Could you check a few things on this model? Use its own coordinates, in mm. A direction names the side the tool comes from. Give positions to 0.01 mm unless a question says otherwise; leave off trailing zeros. Write each loop counter-clockwise with the first axis right and the second up, starting at its lowest first coordinate (ties: lowest second). Pieces come first, ordered by that corner, then holes. Notation, with made-up numbers: (14, -20) - (34, -20) arc R8 ccw to (34, -6) - close; hole circle Ø6 at (-15.75, 62). An arc over 180 degrees is marked (long way). Answer as CSV lines item,"result". Start each with the question number.
Q1. Imagine slicing it at D-D on x = 0. List the corners of the cut face in (y, z) for me.
Q2. Imagine slicing it at A-A on y = 18. List the corners of the cut face in (x, z) for me, and give its area (3 significant figures).
Q3. Imagine slicing it at C-C on x = 7.5. List the corners of the cut face in (y, z) for me.
Q4. Will these pins go through, and if not, where does the flat tip stop? pin 1 Ø2 at (x, z) = (-21, 3.5) entering from +Y; pin 2 Ø10.5 at (x, z) = (-2.5, 2.5) entering from +Y; pin 3 Ø1.5 at (y, z) = (45.25, 7.35) entering from +X; pin 4 Ø2 at (x, z) = (-20, -2.5) entering from +Y.
Q5. We'd pull the mould along X, two halves only. Please class faces 1 (the face through (21.35, 28, 0)), 2 (the face through (-21.35, 29, 0)), 3 (the face through (-20.336, 36.647, 0.055)), 4 (the face through (-14, -1, 0)): pulls with the +X half, pulls with the -X half, needs draft (parallel to the pull), parting line crosses it, or undercut.
Q6. If I drill on line 1 along X through (y, z) = (49, 9); line 2 along Z through (x, y) = (7.5, -0.65); line 3 along X through (y, z) = (-1.2, 5), over which ranges is the centre line in solid material (lowest first)?
Q7. Imagine slicing it at B-B on x = -10. List the corners of the cut face in (y, z) for me.
Q8. On a 3-axis mill with a long thin cutter (end or side, diameter ignored), from which of +Z, -Z, +X, -X, +Y, -Y can I reach the whole of each face in a straight line? I mean faces 5 (the face through (-20.336, 33.843, 6.145)), 6 (the face through (-2.55, -0.99, 2.5)), 7 (the face through (4, 0, -2)). Say none if no direction works.
```python
from build123d import *

# Parameters (mm, degrees)
CROQUIS2_W                  = 152.7
CROQUIS2_H                  = 21
BRIDA_BASE1_DEPTH           = 2
PLIEGUE_START               = -10.5
PLIEGUE_CROQUIZADO1_DEPTH   = 21
PLIEGUE_CROQUIZADO1_2_DEPTH = 21
CROQUIS8_R                  = 1.25
CROQUIS8_R_2                = 3
CORTAR_EXTRUIR1_DEPTH       = 72.000595879
CROQUIS9_R                  = 1.5
CORTAR_EXTRUIR2_DEPTH       = 2


# Read off the part's stored shape, not the designer's step: Pliegue croquizado1
# Sheet-metal steps are written as plain solids
with BuildPart() as part:
    # Croquis2 → Brida base1 (new body)
    with BuildSketch(Plane(origin=(0, 0, 0), x_dir=(1, 0, 0), z_dir=(0, 1, 0))):
        Rectangle(CROQUIS2_W, CROQUIS2_H)
    extrude(amount=-BRIDA_BASE1_DEPTH)

    # Pliegue croquizado1 outline → Pliegue croquizado1 (cut)
    with BuildSketch(Plane.XY.offset(PLIEGUE_START)):
        with BuildLine():
            Line((-76.35, -2), (-18.6134, -2))
            ThreePointArc((-18.6134, -2), (-20.267667209, -1.443395312), (-21.249002398, 0))
            Line((-21.249002398, 0), (-76.35, 0))
            Line((-76.35, 0), (-76.35, -2))
        make_face()
        with BuildLine():
            ThreePointArc((21.249002398, 0), (20.267667209, -1.443395312), (18.6134, -2))
            Line((18.6134, -2), (76.35, -2))
            Line((76.35, -2), (76.35, 0))
            Line((76.35, 0), (21.249002398, 0))
        make_face()
    extrude(amount=PLIEGUE_CROQUIZADO1_DEPTH, mode=Mode.SUBTRACT)

    # Pliegue croquizado1 2 outline → Pliegue croquizado1 2 (add)
    with BuildSketch(Plane.XY.offset(PLIEGUE_START)):
        with BuildLine():
            ThreePointArc((-21.35, 0.7366), (-21.324633029, 0.364854094), (-21.249002398, 0))
            Line((-21.249002398, 0), (-18.6134, 0))
            ThreePointArc((-18.6134, 0), (-19.134254855, 0.215745145), (-19.35, 0.7366))
            Line((-19.35, 0.7366), (-19.35, 55.745355099))
            Line((-19.35, 55.745355099), (-21.35, 55.745355099))
            Line((-21.35, 55.745355099), (-21.35, 0.7366))
        make_face()
        with BuildLine():
            Line((18.6134, 0), (21.249002398, 0))
            ThreePointArc((21.249002398, 0), (21.324633029, 0.364854094), (21.35, 0.7366))
            Line((21.35, 0.7366), (21.35, 55.745355099))
            Line((21.35, 55.745355099), (19.35, 55.745355099))
            Line((19.35, 55.745355099), (19.35, 0.7366))
            ThreePointArc((19.35, 0.7366), (19.134254855, 0.215745145), (18.6134, 0))
        make_face()
    extrude(amount=PLIEGUE_CROQUIZADO1_2_DEPTH)

    # Croquis8 → Cortar-Extruir1 (cut, through all)
    with BuildSketch(Plane(origin=(21.35, 0, 0), x_dir=(0, 0, -1), z_dir=(1, 0, 0))):
        with BuildLine():
            Line((-7, 8.745355099), (-7, 31.745355099))
            ThreePointArc((-7, 31.745355099), (-6.121320344, 33.866675442), (-4, 34.745355099))
            Line((-4, 34.745355099), (-2, 34.745355099))
            Line((-2, 34.745355099), (-2, 5.745355099))
            Line((-2, 5.745355099), (-4, 5.745355099))
            ThreePointArc((-4, 5.745355099), (-6.121320344, 6.624034755), (-7, 8.745355099))
        make_face()
        with BuildLine():
            Line((2, 5.745355099), (4, 5.745355099))
            ThreePointArc((4, 5.745355099), (6.121320344, 6.624034755), (7, 8.745355099))
            Line((7, 8.745355099), (7, 31.745355099))
            ThreePointArc((7, 31.745355099), (6.121320344, 33.866675442), (4, 34.745355099))
            Line((4, 34.745355099), (2, 34.745355099))
            Line((2, 34.745355099), (2, 5.745355099))
        make_face()
        with BuildLine():
            ThreePointArc((0, 55.745355099), (7.424621202, 52.669976301), (10.5, 45.245355099))
            Line((10.5, 45.245355099), (10.5, 55.745355099))
            Line((10.5, 55.745355099), (0, 55.745355099))
        make_face()
        with BuildLine():
            ThreePointArc((-10.5, 45.245355099), (-7.424621202, 52.669976301), (0, 55.745355099))
            Line((0, 55.745355099), (-10.5, 55.745355099))
            Line((-10.5, 55.745355099), (-10.5, 45.245355099))
        make_face()
        with Locations(Location((-7.35, 45.245355099, 0), (0, 0, 90))):
            Circle(CROQUIS8_R)
        with Locations(Location((0, 37.895355099, 0), (0, 0, 90))):
            Circle(CROQUIS8_R)
        with Locations(Location((7.35, 45.245355099, 0), (0, 0, 90))):
            Circle(CROQUIS8_R)
        with Locations(Location((0, 52.595355099, 0), (0, 0, 90))):
            Circle(CROQUIS8_R)
        with Locations(Location((0, 45.245355099, 0), (0, 0, 90))):
            Circle(CROQUIS8_R_2)
    extrude(amount=-CORTAR_EXTRUIR1_DEPTH, mode=Mode.SUBTRACT)

    # Croquis9 → Cortar-Extruir2 (cut)
    with BuildSketch(Plane(origin=(0, 0, 0), x_dir=(1, 0, 0), z_dir=(0, 1, 0))):
        with Locations(Location((-7.5, 5, 0), (0, 0, 270))):
            Circle(CROQUIS9_R)
        with Locations(Location((-7.5, -5, 0), (0, 0, 270))):
            Circle(CROQUIS9_R)
        with Locations(Location((7.5, -5, 0), (0, 0, 90))):
            Circle(CROQUIS9_R)
        with Locations(Location((7.5, 5, 0), (0, 0, 90))):
            Circle(CROQUIS9_R)
        with BuildLine():
            Line((-5, 1.5), (-12.5, 1.5))
            ThreePointArc((-12.5, 1.5), (-14, 0), (-12.5, -1.5))
            Line((-12.5, -1.5), (-5, -1.5))
            ThreePointArc((-5, -1.5), (-2.525126266, -2.525126266), (-1.5, -5))
            ThreePointArc((-1.5, -5), (0, -6.5), (1.5, -5))
            ThreePointArc((1.5, -5), (2.525126266, -2.525126266), (5, -1.5))
            Line((5, -1.5), (12.5, -1.5))
            ThreePointArc((12.5, -1.5), (14, 0), (12.5, 1.5))
            Line((12.5, 1.5), (5, 1.5))
            ThreePointArc((5, 1.5), (2.525126266, 2.525126266), (1.5, 5))
            ThreePointArc((1.5, 5), (0, 6.5), (-1.5, 5))
            ThreePointArc((-1.5, 5), (-2.525126266, 2.525126266), (-5, 1.5))
        make_face()
    extrude(amount=-CORTAR_EXTRUIR2_DEPTH, mode=Mode.SUBTRACT)


solid = part.part
```
Conclusion:
1,outline,"(-2, -10.5) - (0, -10.5) - (0, -6.5) - (-2, -6.5) - close; (-2, 6.5) - (0, 6.5) - (0, 10.5) - (-2, 10.5) - close"
2,outline,"(-21.35, -10.5) - (-19.35, -10.5) - (-19.35, -7) - (-21.35, -7) - close; (-21.35, -2) - (-19.35, -2) - (-19.35, 2) - (-21.35, 2) - close; (-21.35, 7) - (-19.35, 7) - (-19.35, 10.5) - (-21.35, 10.5) - close; (19.35, -10.5) - (21.35, -10.5) - (21.35, -7) - (19.35, -7) - close; (19.35, -2) - (21.35, -2) - (21.35, 2) - (19.35, 2) - close; (19.35, 7) - (21.35, 7) - (21.35, 10.5) - (19.35, 10.5) - close"
2,area,"44.0 mm^2"
3,outline,"(-2, -10.5) - (0, -10.5) - (0, -6.5) - (-2, -6.5) - close; (-2, -3.5) - (0, -3.5) - (0, -1.5) - (-2, -1.5) - close; (-2, 1.5) - (0, 1.5) - (0, 3.5) - (-2, 3.5) - close; (-2, 6.5) - (0, 6.5) - (0, 10.5) - (-2, 10.5) - close"
4,pin 1,"y = 55.44"
4,pin 2,"y = 0"
4,pin 3,"through"
4,pin 4,"y = 55.64"
5,face 1,"pulls with the +X half"
5,face 2,"pulls with the -X half"
5,face 3,"needs draft"
5,face 4,"undercut"
6,line 1,"-21.35 to -19.35, 19.35 to 21.35"
6,line 2,"-10.5 to -6.5, -3.5 to -1.5, 1.5 to 3.5, 6.5 to 10.5"
6,line 3,"-20.55 to -9, -6 to -1.5, 1.5 to 6, 9 to 20.55"
7,outline,"(-2, -10.5) - (0, -10.5) - (0, -1.5) - (-2, -1.5) - close; (-2, 1.5) - (0, 1.5) - (0, 10.5) - (-2, 10.5) - close"
8,face 5,"+X, -X"
8,face 6,"+Y, -Y"
8,face 7,"+Z, -Z, +Y"
